Check sheet for the modelled part. Datum: model origin and axes. Units: mm. Face numbers are marked on the shaded views. A direction names the side the tool comes from. Give positions to 0.01 mm unless a question says otherwise; leave off trailing zeros. Order: outer loops, then holes, each group sorted by start corner. A loop starts at its lowest first (then second) coordinate and runs counter-clockwise, first axis right, second up. Notation, with made-up numbers: (-7.75, -5.75) -> (4.25, -5.75) arc R20 ccw to (4.25, 31.25) -> close; hole circle Ø4 at (9.25, -24). An arc over 180 degrees is marked (long way). Write each question's results on one line, items separated by ' | '.
from build123d import *

# Parameters (mm, degrees)
BASE_FLANGE1_DEPTH         = 64
BREAK_CORNER1_START        = 51
BREAK_CORNER1_DEPTH        = 19
F_9_0_9_DIAMETER_HOLE1_D   = 26
F_10_0_10_DIAMETER_HOLE1_D = 10


# Read off the part's stored shape, not the designer's step: Break-Corner1
# Sheet-metal steps are written as plain solids
with BuildPart() as part:
    # Sketch1 → Base-Flange1 (new body)
    with BuildSketch(Plane.XY):
        with BuildLine():
            Line((0, 0), (0, 35))
            ThreePointArc((0, 35), (10.251262658, 59.748737342), (35, 70))
            Line((35, 70), (102, 70))
            Line((102, 70), (102, 51))
            Line((102, 51), (35, 51))
            ThreePointArc((35, 51), (23.686291501, 46.313708499), (19, 35))
            Line((19, 35), (19, 0))
            Line((19, 0), (0, 0))
        make_face()
    extrude(amount=BASE_FLANGE1_DEPTH)

    # Break-Corner1 outline → Break-Corner1 (cut)
    with BuildSketch(Plane(origin=(0, 0, 0), x_dir=(1, 0, 0), z_dir=(0, 1, 0)).offset(BREAK_CORNER1_START)):
        with BuildLine():
            Line((102, -64), (102, -32))
            ThreePointArc((102, -32), (92.627416998, -54.627416998), (70, -64))
            Line((70, -64), (102, -64))
        make_face()
        with BuildLine():
            ThreePointArc((70, 0), (92.627416998, -9.372583002), (102, -32))
            Line((102, -32), (102, 0))
            Line((102, 0), (70, 0))
        make_face()
    extrude(amount=BREAK_CORNER1_DEPTH, mode=Mode.SUBTRACT)

    # Ø9.0 (9) Diameter Hole1 (through all)
    with Locations(Plane(origin=(70, 70, 32), x_dir=(0, 0, 1), z_dir=(0, 1, 0))):
        with Locations((0, 0)):
            Hole(F_9_0_9_DIAMETER_HOLE1_D / 2)

    # Ø10.0 (10) Diameter Hole1 (through all)
    with Locations(Plane.ZY):
        with Locations((13, 20), (51, 20)):
            Hole(F_10_0_10_DIAMETER_HOLE1_D / 2)


solid = part.part
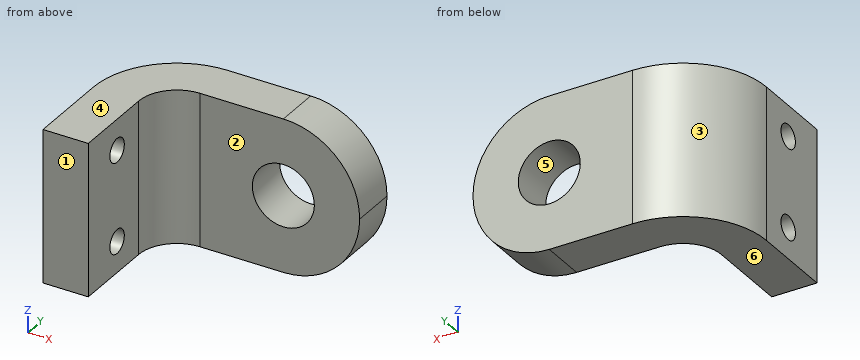
1. Section check B-B on z = 21. Record the cut outline in (x, y), then the cut area to 3 significant figures.
Verdict:
outline: (0, 0) -> (19, 0) -> (19, 35) arc R16 cw to (35, 51) -> (63.07, 51) -> (63.07, 70) -> (35, 70) arc R35 ccw to (0, 35) -> close; (76.93, 51) -> (100.05, 51) -> (100.05, 70) -> (76.93, 70) -> close | area: 2,400 mm^2
2. Mould release check, pull along Z, two halves, no side actions. Record for the marked faces 3, 4, 5 and 6: +Z half, -Z half, draft (parallel to the pull), parting line (faces both ways), or undercut.
Verdict:
face 3: draft | face 4: +Z half | face 5: undercut | face 6: -Z half
3. Access from +Z, -Z, +X, -X, +Y, -Y to the whole of each face (thin tool, end or side, straight path). Record for the marked faces 1 and 2.
Verdict:
face 1: +Z, -Z, +X, -X, -Y | face 2: +Z, -Z, +X, -Y
4. Section check A-A on y = 20. Record the cut outline in (x, z).
Verdict:
outline: (0, 0) -> (19, 0) -> (19, 8) -> (0, 8) -> close; (0, 18) -> (19, 18) -> (19, 46) -> (0, 46) -> close; (0, 56) -> (19, 56) -> (19, 64) -> (0, 64) -> close
5. Section check C-C on x = 62. Record the cut outline in (y, z), then the cut area to 3 significant figures.
Verdict:
outline: (51, 0) -> (70, 0) -> (70, 21.75) -> (51, 21.75) -> close; (51, 42.25) -> (70, 42.25) -> (70, 64) -> (51, 64) -> close | area: 827 mm^2
6. Section check D-D on x = 11.5. Record the cut outline in (y, z), then the cut area to 3 significant figures.
Verdict:
outline: (0, 0) -> (60.94, 0) -> (60.94, 64) -> (0, 64) -> close; hole circle Ø10 at (20, 13); hole circle Ø10 at (20, 51) | area: 3,740 mm^2
7. Gauge pin test, flat ends, axial feed: pin 1 Ø10 at (x, z) = (66, 35) entering from -Y; pin 2 Ø8 at (y, z) = (35.5, 29) entering from +X; pin 3 Ø2 at (y, z) = (39, 49) entering from +X; pin 4 Ø2 at (x, y) = (74.5, 58.5) entering from +Z. Record the tip position at first contact, or that the pin passes through.
Verdict:
pin 1: passes through | pin 2: stops at x = 19.65 | pin 3: stops at x = 19.8 | pin 4: stops at z = 63.81
8. Material ranges on probe 1 along X at (y, z) = (34, 39); probe 2 along Y at (x, z) = (83.5, 31.5); probe 3 along Y at (x, z) = (5.25, 13), recorded low to high. Write a range as from..to.
Verdict:
probe 1: x = 0..19 | probe 2: y = 51..70 | probe 3: y = 0..15, 25..53.44
